Input: dimensioned drawing with shaded views. Units: mm. Origin: part minimum x, y, z. Round coordinates to 2 decimals unless told otherwise and drop trailing zeros. Order: outer loops, then holes, each group sorted by start corner. A loop starts at its lowest first (then second) coordinate and runs counter-clockwise, first axis right, second up.
Item 1: Cut plane A-A on z = 21. Output: boundary loops of the cut face in (x, y), then the cut area to 3 significant figures.
Item 2: Cut plane C-C on x = 2.15. Output: boundary loops of the cut face in (y, z), then the cut area to 4 significant figures.
Item 3: Cut plane B-B on y = 17. Output: boundary loops of the cut face in (x, z), then the cut area to 3 significant figures.
Item 4: Line query: L1, parallel to Y at x = 0.7, z = 86.2; L2, parallel to Y at x = 0.85, z = 21; L3, parallel to Z at x = 1.8, y = 10.5. Output: solid intervals per line, ascending.
Item 5: First-contact query: pin 1 (1.5 mm diameter, centred on x = 2, y = 34.5, fed in from -Z); pin 2 (0.9 mm diameter, centred on x = 2, z = 137.5, fed in from -Y); pin 3 (2 mm diameter, centred on y = 8.5, z = 121, fed in from -X); pin 4 (1.5 mm diameter, centred on x = 1.5, y = 41.5, fed in from +Z). Flat tips, straight axial feed; report the tip coordinate or a pass-through.
Item 6: Cut plane D-D on z = 53. Output: boundary loops of the cut face in (x, y).
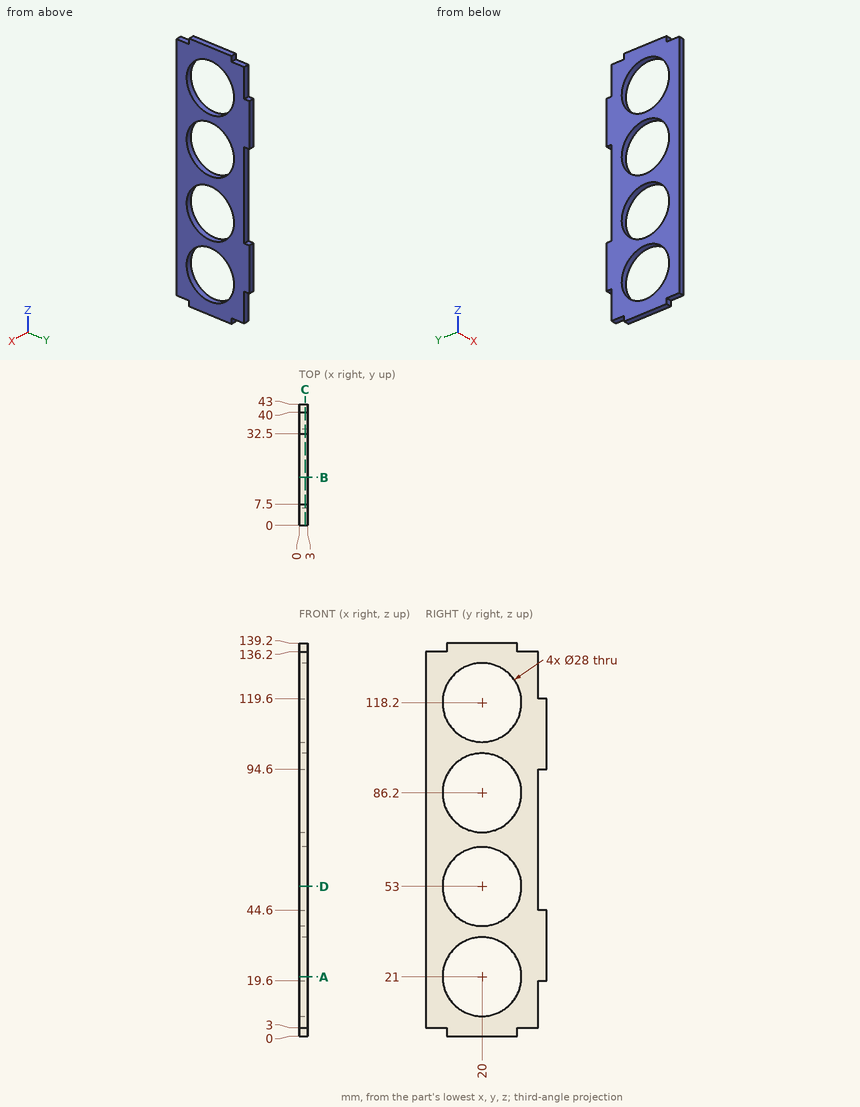
From the geometry:
1. outline: (0, 0) - (3, 0) - (3, 6) - (0, 6) - close; (0, 34) - (3, 34) - (3, 43) - (0, 43) - close
1. area: 45.0 mm2
2. outline: (0, 3) - (7.5, 3) - (7.5, 0) - (32.5, 0) - (32.5, 3) - (40, 3) - (40, 19.6) - (43, 19.6) - (43, 44.6) - (40, 44.6) - (40, 94.6) - (43, 94.6) - (43, 119.6) - (40, 119.6) - (40, 136.2) - (32.5, 136.2) - (32.5, 139.2) - (7.5, 139.2) - (7.5, 136.2) - (0, 136.2) - close; hole circle Ø28 at (20, 21); hole circle Ø28 at (20, 53); hole circle Ø28 at (20, 86.2); hole circle Ø28 at (20, 118.2)
2. area: 3,165 mm2
3. outline: (0, 0) - (3, 0) - (3, 7.33) - (0, 7.33) - close; (0, 34.67) - (3, 34.67) - (3, 39.33) - (0, 39.33) - close; (0, 66.67) - (3, 66.67) - (3, 72.53) - (0, 72.53) - close; (0, 99.87) - (3, 99.87) - (3, 104.53) - (0, 104.53) - close; (0, 131.87) - (3, 131.87) - (3, 139.2) - (0, 139.2) - close
3. area: 89.4 mm2
4. L1: y = 0 to 6, 34 to 40
4. L2: y = 0 to 6, 34 to 43
4. L3: z = 0 to 10.72, 31.28 to 42.72, 63.28 to 75.92, 96.48 to 107.92, 128.48 to 139.2
5. pin 1: stops at z = 3
5. pin 2: stops at y = 7.5
5. pin 3: passes through
5. pin 4: stops at z = 119.6
6. outline: (0, 0) - (3, 0) - (3, 6) - (0, 6) - close; (0, 34) - (3, 34) - (3, 40) - (0, 40) - close
